Build history of the part. All positions in model axes, mm. A direction names the side the tool comes from. Round coordinates to 2 decimals unless told otherwise and drop trailing zeros. Loops run counter-clockwise (first coordinate to the right, second up) from the corner with the lowest first, then second, coordinate; pieces in that order, holes last. Notation, with made-up numbers: (52, 22.25) -> (94, 22.25) arc R35 ccw to (94, 58.25) -> close; hole circle Ø9 at (48.5, 34). An arc over 180 degrees is marked (long way). Put each result on its own line as item: value. Start each with the question number.
Item 1: Cut at B-B, the plane z = 0. List the corners of the cut face in (x, y), plus the area to 3 significant figures.
Item 2: Cut at D-D, the plane x = -38.1. Count the separate pieces of the cut face and the enclosed holes in it, plus the area to 3 significant figures.
Item 3: Tool access for faces 1 (the flat face through (-34, 8.89, 37)), 2 (the flat face through (37, 8.89, 33)), 3 (the flat face through (-32, 4, -50.8)): list every direction of +Z, -Z, +X, -X, +Y, -Y with a clear straight run to the whole face (end or side of a thin tool).
Item 4: Flat gauge pins, fed straight in: pin 1 Ø5.5 at (x, z) = (38.1, 38.1) entering from -Y; pin 2 Ø10 at (y, z) = (10.5, 2.5) entering from +X; pin 3 Ø2 at (x, y) = (13, 3) entering from +Z; pin 4 Ø4 at (x, y) = (-1.5, 2.5) entering from -Z. Where does each tip first touch, or does it go through?
Item 5: Drill centre lines: probe 1 along X at (y, z) = (2.5, -38.1) (3 decimals); probe 2 along X at (y, z) = (11.75, 0); probe 3 along Y at (x, z) = (-24, -41.5). Where is each one in solid material? Low to high. Write a range as [from, to].
Item 6: Pull direction Z, two halves, no side cores. Call faces 4 (the cylindrical face through (48.89, 4.51, 48.99)), 5 (the cylindrical face through (-0.419, 6.791, -31.755)), 6 (the cylindrical face through (-11.59, 15.33, -15.12)): +Z half, -Z half, draft (parallel to the pull), parting line (faces both ways), or undercut.
Item 7: Cut at A-A, the plane y = 1.75. List the corners of the cut face in (x, z) (3 decimals), plus the area to 3 significant figures.
Item 8: Cut at C-C, the plane y = 11.75. List the corners of the cut face in (x, z).
```python
from build123d import *

# Parameters (mm, degrees)
SKETCH1_W           = 101.6
SKETCH1_H           = 101.6
BOSS_EXTRUDE1_DEPTH = 8.89
SKETCH2_R           = 44.45
BOSS_EXTRUDE2_DEPTH = 12.7
FILLET1_R           = 6.35
SKETCH5_R           = 3.175
CUT_EXTRUDE1_DEPTH  = 73.955945611
CHAMFER1_SIZE2      = 18.137479686
CHAMFER1_SIZE       = 12.7
SKETCH6_R           = 19.05
CUT_EXTRUDE2_DEPTH  = 12.7
SKETCH7_R           = 19.05
CUT_EXTRUDE3_DEPTH  = 76.016052282


with BuildPart() as part:
    # Sketch1 → Boss-Extrude1 (new body)
    with BuildSketch(Plane(origin=(0, 0, 0), x_dir=(1, 0, 0), z_dir=(0, 1, 0))):
        Rectangle(SKETCH1_W, SKETCH1_H)
    extrude(amount=BOSS_EXTRUDE1_DEPTH)

    # Sketch2 → Boss-Extrude2 (add)
    with BuildSketch(Plane(origin=(0, 8.89, 0), x_dir=(1, 0, 0), z_dir=(0, 1, 0))):
        with Locations(Location((0, 0, 0), (0, 0, 270))):
            Circle(SKETCH2_R)
    extrude(amount=BOSS_EXTRUDE2_DEPTH)

    # Fillet1
    fillet1_edges = [part.edges().sort_by_distance(p)[0] for p in [
        (-50.8, 4.445, -50.8),
        (50.8, 4.445, -50.8),
        (50.8, 4.445, 50.8),
        (-50.8, 4.445, 50.8),
    ]]
    fillet(fillet1_edges, radius=FILLET1_R)

    # Sketch5 → Cut-Extrude1 (cut, through all)
    with BuildSketch(Plane(origin=(0, 8.89, 0), x_dir=(1, 0, 0), z_dir=(0, 1, 0))):
        with Locations(Location((-38.1, 38.1, 0), (0, 0, 270))):
            Circle(SKETCH5_R)
        with Locations(Location((38.1, 38.1, 0), (0, 0, 270))):
            Circle(SKETCH5_R)
        with Locations(Location((-38.1, -38.1, 0), (0, 0, 270))):
            Circle(SKETCH5_R)
        with Locations(Location((38.1, -38.1, 0), (0, 0, 270))):
            Circle(SKETCH5_R)
    extrude(amount=-CUT_EXTRUDE1_DEPTH, mode=Mode.SUBTRACT)

    # Chamfer1
    chamfer1_edges = [part.edges().sort_by_distance(p)[0] for p in [
        (0, 21.59, -44.45),
    ]]
    chamfer1_side = [part.faces().sort_by_distance(p)[0] for p in [
        (0, 21.336, -44.45),
    ]]
    chamfer(chamfer1_edges, length=CHAMFER1_SIZE - 0.0001, length2=CHAMFER1_SIZE2 - 0.0001, reference=chamfer1_side[0])  # a hair under: the kernel refuses the full size

    # Sketch6 → Cut-Extrude2 (cut)
    with BuildSketch(Plane(origin=(0, 21.59, 0), x_dir=(1, 0, 0), z_dir=(0, 1, 0))):
        with Locations(Location((0, 0, 0), (0, 0, 270))):
            Circle(SKETCH6_R)
    extrude(amount=-CUT_EXTRUDE2_DEPTH, mode=Mode.SUBTRACT)

    # Sketch7 → Cut-Extrude3 (cut, through all)
    with BuildSketch(Plane(origin=(0, 0, 0), x_dir=(1, 0, 0), z_dir=(0, 1, 0))):
        with Locations((-50.8, 0)):
            Circle(SKETCH7_R)
        with Locations((0, 50.8)):
            Circle(SKETCH7_R)
        with Locations((50.8, 0)):
            Circle(SKETCH7_R)
        with Locations((0, -50.8)):
            Circle(SKETCH7_R)
    extrude(amount=CUT_EXTRUDE3_DEPTH, mode=Mode.SUBTRACT)


solid = part.part
```
Reply:
1. outline: (-31.75, 0) -> (31.75, 0) -> (31.75, 17.78) -> (26.31, 21.59) -> (19.05, 21.59) -> (19.05, 8.89) -> (-19.05, 8.89) -> (-19.05, 21.59) -> (-26.31, 21.59) -> (-31.75, 17.78) -> close
1. area: 866 mm^2
2. separate pieces: 4
2. enclosed holes: 0
2. area: 562 mm^2
3. face 1: +Z, -X, +Y
3. face 2: +Z, +X, +Y
3. face 3: -Z, +X, -X, +Y, -Y
4. pin 1: passes through
4. pin 2: stops at x = 33.29
4. pin 3: stops at z = 37.88
4. pin 4: stops at z = -32.07
5. probe 1: x = [-50.8, -41.275], [-34.925, -14.199], [14.199, 34.925], [41.275, 50.8]
5. probe 2: x = [-31.75, -19.05], [19.05, 31.75]
5. probe 3: y = [0, 8.89]
6. face 4: +Z half
6. face 5: -Z half
6. face 6: undercut
7. outline: (-50.8, -44.45) arc R6.35 ccw to (-44.45, -50.8) -> (-19.05, -50.8) arc R19.05 cw to (19.05, -50.8) -> (44.45, -50.8) arc R6.35 ccw to (50.8, -44.45) -> (50.8, -19.05) arc R19.05 cw to (50.8, 19.05) -> (50.8, 44.45) arc R6.35 ccw to (44.45, 50.8) -> (19.05, 50.8) arc R19.05 cw to (-19.05, 50.8) -> (-44.45, 50.8) arc R6.35 ccw to (-50.8, 44.45) -> (-50.8, 19.05) arc R19.05 cw to (-50.8, -19.05) -> close; hole circle Ø6.35 at (-38.1, -38.1); hole circle Ø6.35 at (-38.1, 38.1); hole circle Ø6.35 at (38.1, -38.1); hole circle Ø6.35 at (38.1, 38.1)
7. area: 7,880 mm^2
8. outline: (-37.87, -13.99) arc R40.37 ccw to (-13.99, -37.87) arc R19.05 cw to (13.99, -37.87) arc R40.37 ccw to (37.87, -13.99) arc R19.05 cw to (37.87, 13.99) arc R40.37 ccw to (13.99, 37.87) arc R19.05 cw to (-13.99, 37.87) arc R40.37 ccw to (-37.87, 13.99) arc R19.05 cw to start; hole circle Ø38.1 at (0, 0)
